Check sheet for the modelled part. Datum: model origin and axes. Units: mm. Face numbers are marked on the shaded views. Give positions to 0.01 mm unless a question says otherwise; leave off trailing zeros. Write each loop counter-clockwise with the first axis right and the second up, starting at its lowest first coordinate (ties: lowest second). Pieces come first, ordered by that corner, then holes. Notation, with made-up numbers: (57, 55) -> (106, 55) arc R15 ccw to (106, 70) -> close; hole circle Ø2 at (23.5, 50). An arc over 180 degrees is marked (long way). Answer as a JSON object with one key per item and string values.
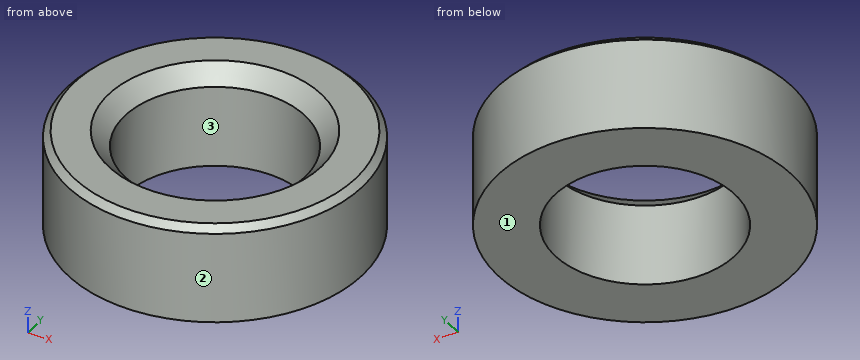
from build123d import *

# Parameters (mm, degrees)
SKETCH014_R     = 4.5
SKETCH014_R_2   = 2.75
PAD007_DEPTH    = 3
CHAMFER001_SIZE = 0.5
CHAMFER002_SIZE = 0.2


with BuildPart() as part:
    # Sketch014 → Pad007 (new body)
    with BuildSketch(Plane.XY):
        Circle(SKETCH014_R)
        Circle(SKETCH014_R_2, mode=Mode.SUBTRACT)
    extrude(amount=PAD007_DEPTH)

    # Chamfer001
    chamfer001_edges = [part.edges().sort_by_distance(p)[0] for p in [
        (-2.75, 0, 3),
    ]]
    chamfer(chamfer001_edges, length=CHAMFER001_SIZE)

    # Chamfer002
    chamfer002_edges = [part.edges().sort_by_distance(p)[0] for p in [
        (-4.5, 0, 3),
    ]]
    chamfer(chamfer002_edges, length=CHAMFER002_SIZE)


with BuildPart() as part_1:
    # Body003 placement: moved
    add(part.part.moved(Location((0, 0, 1))))


solid = part_1.part
1. Sectioned sample at A-A, the plane y = 0. Enter the section's corners in (x, z).
Determined:
{"outline": "(-4.5, 1) -> (-2.75, 1) -> (-2.75, 3.5) -> (-3.25, 4) -> (-4.3, 4) -> (-4.5, 3.8) -> close; (2.75, 1) -> (4.5, 1) -> (4.5, 3.8) -> (4.3, 4) -> (3.25, 4) -> (2.75, 3.5) -> close"}
2. Go/stop test with flat-tipped pins: P1, Ø1, axis at y = -3.5, z = 2.5, coming from the -X side; P2, Ø1, axis at y = 2.5, z = 3, coming from the +X side. Record where each tip stops, or that it passes through.
Determined:
{"P1": "x = -3.35", "P2": "x = 4.03"}
3. Scan lines: L1, parallel to Y at x = 0, z = 1.85; L2, parallel to X at y = 2, z = 3.3; L3, parallel to Y at x = 1.25, z = 3.3. Record each from-to range of solid material in increasing order. Write a range as [from, to].
Determined:
{"L1": "[-4.5, -2.75], [2.75, 4.5]", "L2": "[-4.03, -1.89], [1.89, 4.03]", "L3": "[-4.32, -2.45], [2.45, 4.32]"}
4. Mould release check, pull along Y, two halves, no side actions. Record for the marked faces 1, 2 and 3: released by +Y, released by -Y, zero draft, split by the parting line, or undercut.
Determined:
{"face 1": "zero draft", "face 2": "split by the parting line", "face 3": "undercut"}
5. Sectioned sample at C-C, the plane z = 2.2. Enter the section's corners in (x, y).
Determined:
{"outline": "circle Ø9 at (0, 0); hole circle Ø5.5 at (0, 0)"}
